The listing builds one solid part. Answer for the finished solid, in the listing's coordinates (mm). Give positions to 0.01 mm unless a question says otherwise; leave off trailing zeros. Write each loop counter-clockwise with the first axis right and the second up, starting at its lowest first coordinate (ties: lowest second). Pieces come first, ordered by that corner, then holes. Notation, with made-up numbers: (6.25, 79.25) - (45.25, 79.25) arc R8 ccw to (45.25, 84.25) - close; hole circle Ø8 at (75, -6). An arc over 180 degrees is marked (long way). Return JSON: item names as keys, results as strings.
from build123d import *

# Parameters (mm, degrees)
F0_R     = 19.05
F1_DEPTH = 6.35
F4_DEPTH = 159.5317363987
F5_R     = 5.08


with BuildPart() as f1:
    # F0 (on Front) → F1 (new body)
    with BuildSketch(Plane.XZ):
        with BuildLine():
            Line((0, 46.5095229447), (0, 0))
            Line((0, 0), (114.3, 0))
            Line((114.3, 0), (114.3, 110.7982022234))
            Line((114.3, 110.7982022234), (0, 152.4))
            Line((0, 152.4), (0, 49.8115229447))
            Line((0, 49.8115229447), (10.16, 49.8115229447))
            ThreePointArc((10.16, 49.8115229447), (11.811, 48.1605229447), (10.16, 46.5095229447))
            Line((10.16, 46.5095229447), (0, 46.5095229447))
        make_face()
        with Locations((40.64, 85.09)):
            Circle(F0_R, mode=Mode.SUBTRACT)
    extrude(amount=F1_DEPTH)

    # F3 (on face) → F4 (cut, through all)
    with BuildSketch(Plane(origin=(-48.9804158581, 0, 17.8274134343), x_dir=(0, -1, 0), z_dir=(-0.9396926208, 0, 0.3420201433))):
        Polygon((6.35, 143.2091554078), (0, 143.2091554078), (6.35, 140.2481017785), align=None)
    extrude(amount=-F4_DEPTH, mode=Mode.SUBTRACT)

    # F5
    f5_edges = [f1.edges().sort_by_distance(p)[0] for p in [
        (0, -3.175, 150.824456),
        (114.3, -3.175, 109.222658),
        (114.3, -3.175, 0),
        (0, -3.175, 0),
    ]]
    fillet(f5_edges, radius=F5_R)


solid = f1.part
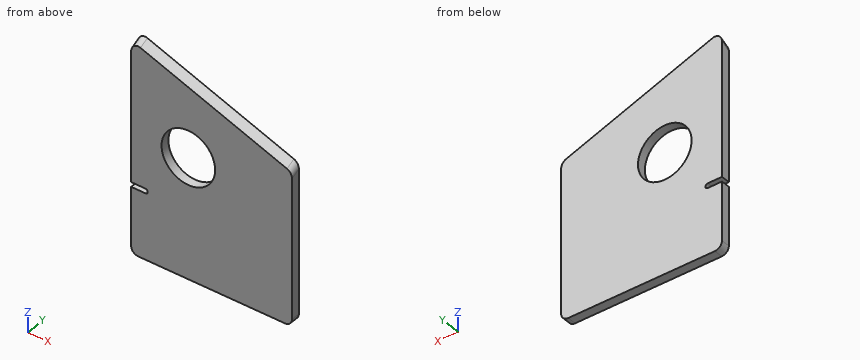
Item 1: A cutting plane is placed at B-B on x = 46. Determine the outline of the cut face in (y, z), then the cut area to 3 significant figures.
Answer below:
{"outline": "(-6.35, 0) - (0, 0) - (0, 66.81) - (-6.35, 66.81) - close; (-6.35, 103.37) - (0, 103.37) - (0, 135.66) - (-6.35, 132.51) - close", "area": "619 mm²"}
Item 2: A cutting plane is placed at C-C on x = 15. Determine the outline of the cut face in (y, z).
Answer below:
{"outline": "(-6.35, 0) - (0, 0) - (0, 146.94) - (-6.35, 143.79) - close"}
Item 3: A flat-ended cylindrical pin translates along its axis: P1, Ø1.9, axis at x = 4.5, y = -4, coming from the +Z side. Find the tip coordinate at first contact, or state that the pin passes through.
Answer below:
{"P1": "stops at z = 148.72"}
Item 4: A cutting plane is placed at A-A on z = 85.09. Determine the outline of the cut face in (x, y).
Answer below:
{"outline": "(0, -6.35) - (21.59, -6.35) - (21.59, 0) - (0, 0) - close; (59.69, -6.35) - (114.3, -6.35) - (114.3, 0) - (59.69, 0) - close"}
Item 5: Consider L1, parallel to Z at x = 40.64, y = -3; L2, parallel to Z at x = 51, y = -2.5; L3, parallel to X at y = -4.5, z = 90.5. Determine where each line is inside the solid, lowest interval first.
Answer below:
{"L1": "z = 0 to 66.04, 104.14 to 136.12", "L2": "z = 0 to 69.1, 101.08 to 132.6", "L3": "x = 0 to 22.37, 58.91 to 114.3"}
Item 6: A cutting plane is placed at D-D on x = 68. Determine the outline of the cut face in (y, z).
Answer below:
{"outline": "(-6.35, 0) - (0, 0) - (0, 127.65) - (-6.35, 124.5) - close"}
